Input: part model. Units: mm. Frame: model coordinates. A direction names the side the tool comes from. Round coordinates to 2 decimals unless told otherwise and drop trailing zeros. Loops run counter-clockwise (first coordinate to the right, second up) from the corner with the lowest first, then second, coordinate; pieces in that order, holes last.
1) Section A-A, the plane z = 0. Return loops of the section in (x, y) (3 decimals).
2) Draft query along Y for faces 3 (the face through (193.675, -11, 0)), 4 (the face through (193.675, 0, 0)), 5 (the face through (198.5, -1.26, -3.05)), 6 (the face through (199, -9.423, 0)). Return one class per face: pulls with the +Y half, pulls with the -Y half, needs draft (parallel to the pull), parting line crosses it, or undercut.
3) Ray query, line 1 along Z through (x, y) = (199.5, 0); line 2 along Y through (x, z) = (199.5, 0); line 3 along X through (y, z) = (-2, -2.5) (3 decimals). Return the intervals inside material, ascending.
4) Section C-C, the plane y = -6.5. Return loops of the section in (x, z), and give its area (3 significant figures).
5) Access query for faces 1 (the face through (0, 0, 0)), 2 (the face through (199, 9.423, 0)). Directions: +Z, -Z, +X, -X, +Y, -Y. A direction counts if a zero-diameter tool reaches every point of the face in a straight line with its end or side. Return the directions, or none.
6) Section B-B, the plane x = 88.5. Return loops of the section in (y, z).
7) First-contact query: pin 1 (7.5 mm diameter, centred on x = 200.5, z = 3, fed in from -Y); pin 2 (6 mm diameter, centred on y = 0, z = 0, fed in from +X) (3 decimals); pin 3 (12 mm diameter, centred on x = 85, z = 8, fed in from -Y). Flat tips, straight axial feed; report the tip coordinate or a pass-through.
Autodesk Inventor part; units mm, degrees
ref_plane "YZ Plane" through (0, 0, 0) normal (1, 0, 0) x (0, 1, 0)
ref_plane "XZ Plane" through (0, 0, 0) normal (0, 1, 0) x (-1, 0, 0)
ref_plane "XY Plane" through (0, 0, 0) normal (0, 0, 1) x (1, 0, 0)
sketch "Sketch1" plane through (0, 0, 0) normal (1, 0, 0) x (0, 1, 0)
  circle A0 centre (0, 0) radius 12.7
  dimension "d0" = 25.4
extrude "Extrusion1" add sketch "Sketch1" along normal blind 203.2
sketch "Sketch2" plane through (203.2, 0, 0) normal (1, 0, 0) x (0, 0, -1)
  circle A0 centre (0, 0) radius 12.7
  circle A1 centre (0, 0) radius 12.7
  line L0 (-8.5141, 9.4234) -> (8.5141, 9.4234)
  line L1 (-8.5141, -9.4234) -> (8.5141, -9.4234)
  line L2 (-17.78, 0) -> (17.78, 0)
  line L3 (0, -17.78) -> (0, 17.78)
  circle A2 centre (0, 0) radius 3.302
  dimension "d3" = 18.8468
  dimension "d4" = 6.604
extrude "Extrusion2" cut sketch "Sketch2" against normal blind 9.525 contours L0 L3 A0 | A0 L3 L1 | A2 L3 L2 | L2 L3 A2 | L3 L0 A0 | A0 L1 L3 | L3 A2 L2 | L2 A2 L3
properties part number "DART Rod"
Final values:
1. outline: (0, -12.7) - (193.675, -12.7) - (193.675, -9.423) - (203.2, -9.423) - (203.2, -3.302) - (193.675, -3.302) - (193.675, 3.302) - (203.2, 3.302) - (203.2, 9.423) - (193.675, 9.423) - (193.675, 12.7) - (0, 12.7) - close
2. face 3: needs draft
2. face 4: undercut
2. face 5: undercut
2. face 6: pulls with the -Y half
3. line 1: z = -12.7 to -3.3, 3.3 to 12.7
3. line 2: y = -9.42 to -3.3, 3.3 to 9.42
3. line 3: x = 0 to 193.675
4. outline: (0, -10.91) - (203.2, -10.91) - (203.2, 10.91) - (0, 10.91) - close
4. area: 4,430 mm2
5. face 1: +Z, -Z, -X, +Y, -Y
5. face 2: +Z, -Z, +X, +Y
6. outline: circle Ø25.4 at (0, 0)
7. pin 1: stops at y = -9.42
7. pin 2: stops at x = 193.675
7. pin 3: stops at y = -12.54
